```python
from build123d import *

# Parameters (mm, degrees)
BOX_W                = 7.5
BOX_H                = 8.8
BOX_DEPTH            = 5.9
BOX001_W             = 10
BOX001_H             = 10
BOX001_DEPTH         = 1.8
BOX002_W             = 3.1
BOX002_H             = 7.9
BOX002_DEPTH         = 3.3
BOX003_W             = 2.3
BOX003_H             = 1.4
BOX003_DEPTH         = 1.5
BOX004_W             = 10
BOX004_H             = 10
BOX004_DEPTH         = 2.6
BODY_PITCH_ANGLE     = -90
BODY_PLACEMENT_ANGLE = -90


with BuildPart() as part:
    # Box → Box (join)
    with BuildSketch(Plane.XY.offset(-0.6)):
        with Locations((3.75, 4.4)):
            Rectangle(BOX_W, BOX_H)
    extrude(amount=BOX_DEPTH)

    # Box001 → Box001 (cut)
    with BuildSketch(Plane(origin=(1.5, 0, 1), x_dir=(1, 0, 0), z_dir=(0, 0, 1))):
        with Locations((5, 5)):
            Rectangle(BOX001_W, BOX001_H)
    extrude(amount=BOX001_DEPTH, mode=Mode.SUBTRACT)

    # Box002 → Box002 (cut)
    with BuildSketch(Plane(origin=(3.8, 0.45, 1), x_dir=(1, 0, 0), z_dir=(0, 0, 1))):
        with Locations((1.55, 3.95)):
            Rectangle(BOX002_W, BOX002_H)
    extrude(amount=BOX002_DEPTH, mode=Mode.SUBTRACT)

    # Box003 → Box003 (cut)
    with BuildSketch(Plane(origin=(1.5, 3.7, 2.8), x_dir=(1, 0, 0), z_dir=(0, 0, 1))):
        with Locations((1.15, 0.7)):
            Rectangle(BOX003_W, BOX003_H)
    extrude(amount=BOX003_DEPTH, mode=Mode.SUBTRACT)

    # Box004 → Box004 (cut)
    with BuildSketch(Plane(origin=(3.8, 0, 1), x_dir=(1, 0, 0), z_dir=(0, 0, 1))):
        with Locations((5, 5)):
            Rectangle(BOX004_W, BOX004_H)
    extrude(amount=BOX004_DEPTH, mode=Mode.SUBTRACT)


with BuildPart() as part_1:
    # Body pitch: moved
    add(part.part.rotate(Axis((0, 0, 0), (0, 1, 0)), BODY_PITCH_ANGLE))


with BuildPart() as part_2:
    # Body placement: moved
    add(part_1.part.rotate(Axis((0, 0, 0), (0, 0, 1)), BODY_PLACEMENT_ANGLE))


solid = part_2.part
```
The model under review builds one solid part; all positions refer to its coordinate system, in mm. A direction names the side the tool comes from. Give positions to 0.01 mm unless a question says otherwise; leave off trailing zeros. Write each loop counter-clockwise with the first axis right and the second up, starting at its lowest first coordinate (ties: lowest second). Pieces come first, ordered by that corner, then holes. Notation, with made-up numbers: M 65,29 L 112,29 A19 cw 112,42 Z; hole C -23,-35.5 d4. An arc over 180 degrees is marked long. Write item = value, one per line. Start each with the question number.
Q1. We need section D-D (y = 2.15). State the section outline as (x, z) points.
Q2. We need section B-B (x = 3). State the section outline as (y, z) points.
Q3. We need section A-A (z = 6.75). State the section outline as (x, y) points, plus the area to 3 significant figures.
Q4. For line 1 (Y direction, x = 3.75, z = 6); line 2 (Y direction, x = 1.75, z = 2); line 3 (X direction, y = 3.7, z = 4.5), list the stretches that pass through material, from the lowest coordinate up.
Q5. Machinability: for faces 4 (the face through (0, 3, 3)), 5 (the face through (2, 4, 3.8)), 6 (the face through (7, 2.8, 3)), which of the approach directions +Z, -Z, +X, -X, +Y, -Y give a long, thin tool a straight path to every point of the face, cutting with its end or side? Answer none if there is none.
Q6. We need section C-C (z = 2). State the section outline as (x, y) points, plus the area to 3 significant figures.
Q7. Mouldability with a two-part tool opening along X and no side actions: class faces 1 (the face through (4, 1, 4)), 2 (the face through (5.1, 4, 3)), 3 (the face through (8.8, 3, 3)) as released by +X, released by -X, zero draft, split by the parting line, or undercut.
Result set:
q1.outline = M 0,0 L 8.8,0 L 8.8,1.5 L 0,1.5 Z
q2.outline = M -0.6,0 L 5.3,0 L 5.3,7.5 L 3.6,7.5 L 3.6,6.9 L 4.3,6.9 L 4.3,3.8 L 2.8,3.8 L 2.8,1.5 L 1,1.5 L 1,7.5 L -0.6,7.5 Z
q3.outline = M 0,-0.6 L 8.8,-0.6 L 8.8,1 L 0,1 Z; M 0,3.6 L 0.45,3.6 L 0.45,4.3 L 8.35,4.3 L 8.35,3.6 L 8.8,3.6 L 8.8,5.3 L 0,5.3 Z
q3.area = 23.5 mm2
q4.line_1 = -0.6 to 1, 4.3 to 5.3
q4.line_2 = -0.6 to 1, 2.8 to 5.3
q4.line_3 = 0 to 0.45, 8.35 to 8.8
q5.face_4 = +Z, -Z, -X, +Y, -Y
q5.face_5 = none
q5.face_6 = +Z, +X, -X
q6.outline = M 0,-0.6 L 8.8,-0.6 L 8.8,1 L 0,1 Z; M 0,2.8 L 3.7,2.8 L 3.7,4.3 L 5.1,4.3 L 5.1,2.8 L 8.8,2.8 L 8.8,5.3 L 0,5.3 Z
q6.area = 34.0 mm2
q7.face_1 = zero draft
q7.face_2 = undercut
q7.face_3 = released by +X
